The drawing under review shows one solid part. Ordinate dimensions are in mm from its lowest x, y, z. Coordinates: 2 decimals unless noted, no trailing zeros. Write each loop counter-clockwise with the first axis right and the second up, starting at its lowest first coordinate (ties: lowest second). Pieces come first, ordered by that corner, then holes.
1) Add section A-A, the plane z = 0.5. State the section outline as (x, y) points, then the cut area to 3 significant figures.
2) For line 1 (X direction, y = 5, z = 0.8); line 2 (Y direction, x = 38.5, z = 0.65) (1 decimal); line 3 (X direction, y = 61, z = 1.15) (1 decimal), list the stretches that pass through material, from the lowest coordinate up.
3) For P1, Ø0.6, axis at y = 30.5, z = 1, coming from the -X side; P2, Ø3, axis at x = 5, y = 60, coming from the +Z side; P3, Ø1, axis at y = 36, z = 1, coming from the +X side, all flat-tipped, find the tip position at first contact; note any pin that passes through.
4) Add section B-B, the plane y = 33. State the section outline as (x, z) points.
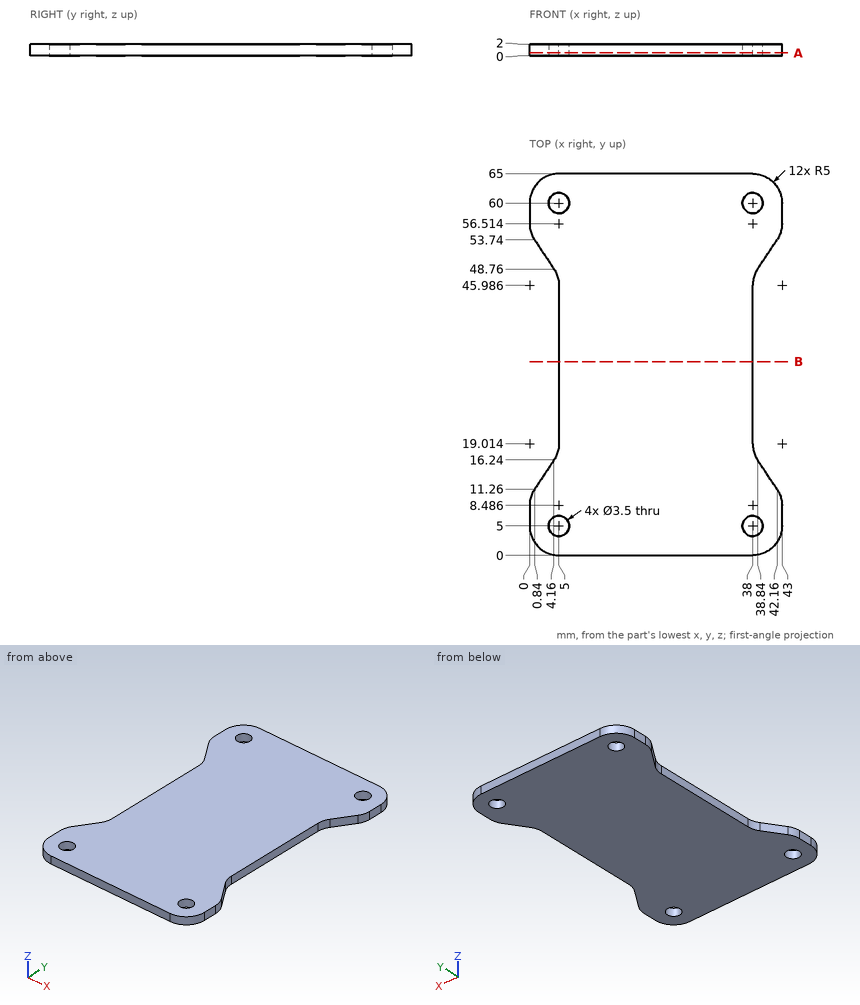
Geometry results:
1. outline: (0, 5) arc R5 ccw to (5, 0) - (38, 0) arc R5 ccw to (43, 5) - (43, 8.49) arc R5 ccw to (42.16, 11.26) - (38.84, 16.24) arc R5 cw to (38, 19.01) - (38, 45.99) arc R5 cw to (38.84, 48.76) - (42.16, 53.74) arc R5 ccw to (43, 56.51) - (43, 60) arc R5 ccw to (38, 65) - (5, 65) arc R5 ccw to (0, 60) - (0, 56.51) arc R5 ccw to (0.84, 53.74) - (4.16, 48.76) arc R5 cw to (5, 45.99) - (5, 19.01) arc R5 cw to (4.16, 16.24) - (0.84, 11.26) arc R5 ccw to (0, 8.49) - close; hole circle Ø3.5 at (5, 5); hole circle Ø3.5 at (5, 60); hole circle Ø3.5 at (38, 5); hole circle Ø3.5 at (38, 60)
1. area: 2,360 mm2
2. line 1: x = 0 to 3.25, 6.75 to 36.25, 39.75 to 43
2. line 2: y = 0 to 3.3, 6.7 to 16.8, 48.2 to 58.3, 61.7 to 65
2. line 3: x = 0.1 to 3.6, 6.4 to 36.6, 39.4 to 42.9
3. P1: stops at x = 5
3. P2: passes through
3. P3: stops at x = 38
4. outline: (5, 0) - (38, 0) - (38, 2) - (5, 2) - close
